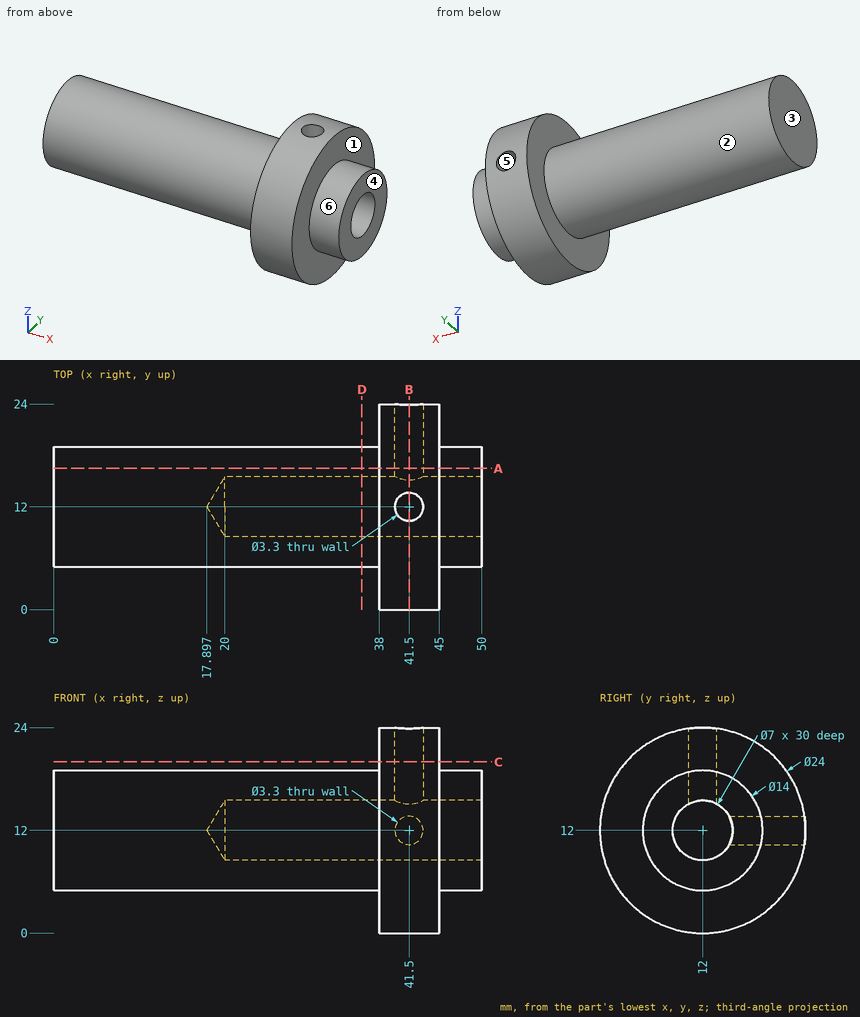
Answer from the drawing. Dimensions are ordinates in mm from the lowest x, y and z of the part. A direction names the side the tool comes from. Coordinates: 2 decimals unless noted, no trailing zeros. Loops run counter-clockwise (first coordinate to the right, second up) from the corner with the lowest first, then second, coordinate; pieces in that order, holes last. Notation, with made-up numbers: (14, 64.25) -> (44, 64.25) arc R37 cw to (44, 102.25) -> close; hole circle Ø7 at (-1, -5). An arc over 180 degrees is marked (long way). Answer as CSV lines item,"result".
Q1. The part is cut by section B-B on x = 41.5. Write down the section's boundary in (y, z), and give its area (3 significant figures).
Findings:
outline,"(10.35, 15.09) -> (10.35, 23.89) arc R12 ccw (long way) to (23.89, 10.35) -> (15.09, 10.35) arc R3.5 cw (long way) to start; (13.65, 15.09) arc R3.5 cw to (15.09, 13.65) -> (23.89, 13.65) arc R12 ccw to (13.65, 23.89) -> close"
area,"357 mm²"
Q2. A tool of negligible diameter and unlimited length cuts with its end or side. For the marked faces 1, 2 and 3, from which of +Z, -Z, +X, -X, +Y, -Y can it reach the whole face along a straight path? Write none if from no direction.
Findings:
face 1,"+X"
face 2,"-X"
face 3,"+Z, -Z, -X, +Y, -Y"
Q3. The part is cut by section A-A on y = 16.5. Write down the section's boundary in (x, z).
Findings:
outline,"(0, 6.64) -> (38, 6.64) -> (38, 0.88) -> (45, 0.88) -> (45, 6.64) -> (50, 6.64) -> (50, 17.36) -> (45, 17.36) -> (45, 23.12) -> (38, 23.12) -> (38, 17.36) -> (0, 17.36) -> close; hole circle Ø3.3 at (41.5, 12)"
Q4. Find the intervals of material crossed by probe 1 along X at (y, z) = (10.75, 4.5); probe 2 along Y at (x, z) = (42.5, 12); probe 3 along Z at (x, y) = (41, 17), in increasing order.
Findings:
probe 1,"x = 38 to 45"
probe 2,"y = 0 to 8.5"
probe 3,"z = 1.09 to 10.43, 13.57 to 22.91"
Q5. For a pull along X with two mould halves and no side action, classify the marked faces 4, 5 and 6 as +X half, -X half, draft (parallel to the pull), parting line (faces both ways), or undercut.
Findings:
face 4,"+X half"
face 5,"undercut"
face 6,"draft"
Q6. The part is cut by section D-D on x = 36. Write down the section's boundary in (y, z), and give its area (3 significant figures).
Findings:
outline,"circle Ø14 at (12, 12); hole circle Ø7 at (12, 12)"
area,"115 mm²"
Q7. Each of these flat-tipped pins is pushed along its axis until it touches: pin 1 (5 mm diameter, centred on x = 7, z = 16, fed in from +Y); pin 2 (8 mm diameter, centred on x = 34.5, z = 2.5, fed in from -Y); pin 3 (4 mm diameter, centred on x = 24.5, y = 11, fed in from -Z). Where does it stop, or does it pass through?
Findings:
pin 1,"stops at y = 18.84"
pin 2,"stops at y = 2.68"
pin 3,"stops at z = 5"
Q8. The part is cut by section C-C on z = 20. Write down the section's boundary in (x, y).
Findings:
outline,"(38, 3.06) -> (45, 3.06) -> (45, 20.94) -> (38, 20.94) -> close; hole circle Ø3.3 at (41.5, 12)"
